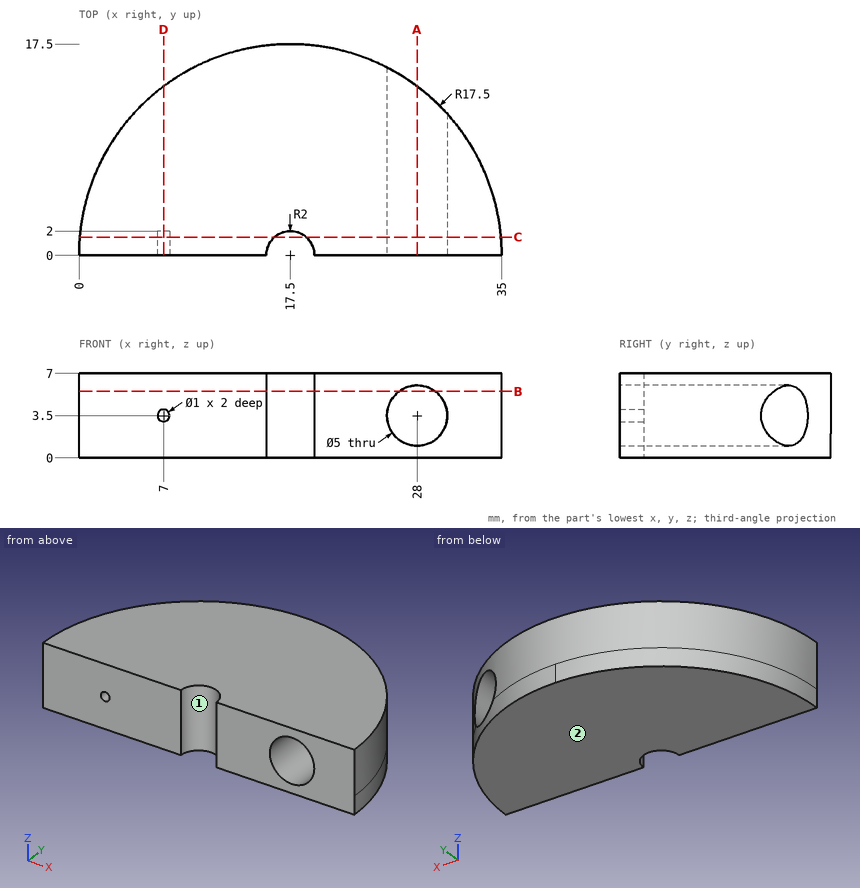
Geometry: see drawing. Coordinates: mm, zero at the bounding-box minimum. Round coordinates to 2 decimals unless told otherwise and drop trailing zeros. Loops run counter-clockwise (first coordinate to the right, second up) from the corner with the lowest first, then second, coordinate; pieces in that order, holes last. Notation, with made-up numbers: (-17.75, 75.5) -> (23.25, 75.5) arc R20 ccw to (23.25, 90.5) -> close; hole circle Ø1 at (63, 2.25). An arc over 180 degrees is marked (long way). Use one line per item in the form item = value. Start each with the question number.
Item 1: Contact query for flat-ended pins moving along their axis: pin 1 Ø3 at (x, z) = (24, 5) entering from +Y; pin 2 Ø3 at (y, z) = (8.5, 6) entering from +X; pin 3 Ø0.8 at (x, z) = (7, 3.5) entering from -Y. Output: stop coordinate, or through.
Item 2: Material intervals for L1, parallel to X at y = 0.85, z = 3.5; L2, parallel to X at y = 0.45, z = 3.5; L3, parallel to Y at x = 25.5, z = 1.5, sorted ascending. Write a range as from..to.
Item 3: Section query C-C on y = 1.5. Return the cut outline in (x, z).
Item 4: Section query B-B on z = 5.5. Return the cut outline in (x, y).
Item 5: Mould query, pull axis X, two halves, no side actions, for the marked faces 1 and 2. Classes: pulls with the +X half, pulls with the -X half, needs draft (parallel to the pull), parting line crosses it, or undercut.
Item 6: Section query D-D on x = 7. Return the cut outline in (y, z), then the cut area to 3 significant figures.
Item 7: Section query A-A on x = 28. Return the cut outline in (y, z).
Ans:
q1.pin_1 = 16.77
q1.pin_2 = 33.54
q1.pin_3 = 2
q2.L1 = 0.02..6.5, 7.5..15.69, 19.31..25.5, 30.5..34.98
q2.L2 = 0.01..6.5, 7.5..15.55, 19.45..25.5, 30.5..34.99
q2.L3 = 0..15.56
q3.outline = (0.06, 0) -> (16.18, 0) -> (16.18, 7) -> (0.06, 7) -> close; (18.82, 0) -> (34.94, 0) -> (34.94, 7) -> (18.82, 7) -> close; hole circle Ø1 at (7, 3.5); hole circle Ø5 at (28, 3.5)
q4.outline = (0, 0) -> (15.5, 0) arc R2 cw to (19.5, 0) -> (26.5, 0) -> (26.5, 15.01) arc R17.5 ccw to start; (29.5, 0) -> (35, 0) arc R17.5 ccw to (29.5, 12.74) -> close
q5.face_1 = undercut
q5.face_2 = needs draft
q6.outline = (0, 0) -> (14, 0) -> (14, 7) -> (0, 7) -> (0, 4) -> (2, 4) -> (2, 3) -> (0, 3) -> close
q6.area = 96.0 mm^2
q7.outline = (0, 0) -> (14, 0) -> (14, 1) -> (0, 1) -> close; (0, 6) -> (14, 6) -> (14, 7) -> (0, 7) -> close
